CAD build for the part. Positions are in the model's coordinates, mm. Face numbers are marked on the shaded views. A direction names the side the tool comes from. Coordinates: 2 decimals unless noted, no trailing zeros. Loops run counter-clockwise (first coordinate to the right, second up) from the corner with the lowest first, then second, coordinate; pieces in that order, holes last. Notation, with made-up numbers: M 29.25,-15.75 L 37.25,-15.75 A28 cw 37.25,11.25 Z; hole C 65.5,66.25 d4. An arc over 180 degrees is marked long. Answer as a JSON object with one key per item and string values. Group by question number.
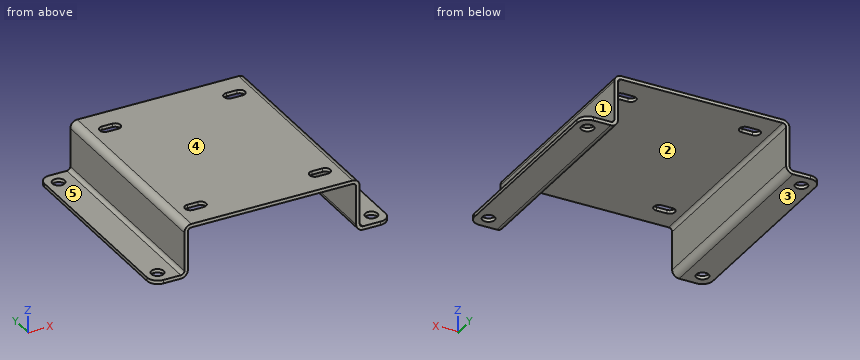
Autodesk Inventor part; units mm, degrees
ref_plane "YZ Plane" through (0, 0, 0) normal (1, 0, 0) x (0, 1, 0)
ref_plane "XZ Plane" through (0, 0, 0) normal (0, 1, 0) x (-1, 0, 0)
ref_plane "XY Plane" through (0, 0, 0) normal (0, 0, 1) x (1, 0, 0)
sketch "Sketch1" plane through (0, 0, 0) normal (0, 0, 1) x (1, 0, 0)
  line L0 (-50, -60) -> (50, -60)
  line L1 (50, -60) -> (50, 60)
  line L2 (50, 60) -> (-50, 60)
  line L3 (-50, 60) -> (-50, -60)
  line L4 (-50, -60) -> (50, 60) construction
  line L5 (50, -60) -> (-50, 60) construction
  point P0 (0, 0)
  dimension "d0" = 100
  dimension "d1" = 120
extrude "Plate1" add sketch "Sketch1" along normal blind 2
sketch "Sketch5" plane through (48, -60, 2) normal (1, 0, 0) x (0, 1, 0)
  line L0 (120, 0) -> (0, 0)
  line L1 (0, 0) -> (0, -30)
  line L2 (0, -30) -> (120, -30)
  line L3 (120, -30) -> (120, 0)
edge flange "Flange2" height 30 angle 90 thickness 2 bend radius 2 thickness toward (1, 0, 0) relief tear relief width 2 relief depth 1 corner gap 2 corner form 0 edges at (50, 0, 0) (-50, 0, 0) wall of the first edge with corners at (48, 60, 2) (48, -60, 2) (48, -60, -28) (48, 60, -28)
bend "Bend2"
corner "Corner2"
sketch "Sketch6" plane through (-48, -60, -26) normal (0, 0, -1) x (-1, 0, 0)
  line L0 (0, 120) -> (0, 0)
  line L1 (0, 0) -> (20, 0)
  line L2 (20, 0) -> (20, 120)
  line L3 (20, 120) -> (0, 120)
edge flange "Flange3" height 20 angle 90 thickness 2 bend radius 2 thickness toward (0, 0, -1) relief tear relief width 2 relief depth 1 corner gap 2 corner form 0 edges at (-50, 0, -28) (50, 0, -28) wall of the first edge with corners at (-48, 60, -26) (-48, -60, -26) (-68, -60, -26) (-68, 60, -26)
bend "Bend3"
corner "Corner3"
sketch "Sketch7" plane through (0, 0, 2) normal (0, 0, 1) x (1, 0, 0)
  line L0 (-38.5, 45) -> (-32.5, 45) construction
  line L1 (-38.5, 48) -> (-32.5, 48)
  line L2 (-32.5, 42) -> (-38.5, 42)
  arc A0 (-38.5, 48) -> (-38.5, 42) centre (-38.5, 45) ccw
  arc A1 (-32.5, 42) -> (-32.5, 48) centre (-32.5, 45) ccw
  line L3 (0, 0) -> (0, 36.7508)
  line L4 (0, 0) -> (-25.7119, 0)
  line L5 (32.5, 45) -> (38.5, 45) construction
  line L6 (32.5, 48) -> (38.5, 48)
  line L7 (38.5, 42) -> (32.5, 42)
  arc A2 (32.5, 48) -> (32.5, 42) centre (32.5, 45) ccw
  arc A3 (38.5, 42) -> (38.5, 48) centre (38.5, 45) ccw
  line L8 (-38.5, -45) -> (-32.5, -45) construction
  line L9 (-38.5, -42) -> (-32.5, -42)
  line L10 (-32.5, -48) -> (-38.5, -48)
  arc A4 (-38.5, -42) -> (-38.5, -48) centre (-38.5, -45) ccw
  arc A5 (-32.5, -48) -> (-32.5, -42) centre (-32.5, -45) ccw
  line L11 (32.5, -45) -> (38.5, -45) construction
  line L12 (32.5, -42) -> (38.5, -42)
  line L13 (38.5, -48) -> (32.5, -48)
  arc A6 (32.5, -42) -> (32.5, -48) centre (32.5, -45) ccw
  arc A7 (38.5, -48) -> (38.5, -42) centre (38.5, -45) ccw
  point P0 (-35.5, 45)
  point P1 (35.5, 45)
  point P2 (-35.5, -45)
  point P3 (35.5, -45)
  dimension "d42" = 6
  dimension "d43" = 6
  dimension "d50" = 71
  dimension "d51" = 90
extrude "Cut1" cut sketch "Sketch7" against normal blind 2
sketch "Sketch8" plane through (-68, -60, -26) normal (0, 0, 1) x (1, 0, 0)
  circle A0 centre (7, 112) radius 3.5
  circle A1 centre (7, 8) radius 3.5
  line L0 (16, 120) -> (0, 120)
  line L1 (0, 120) -> (0, 0)
  line L2 (0, 60) -> (53.6667, 60)
  point P0 (68, 60)
  dimension "d54" = 7
  dimension "d55" = 8
  dimension "d56" = 7
extrude "Cut2" cut sketch "Sketch8" against normal blind 2
mirror "Mirror1" about plane through (0, 0, 0) normal (1, 0, 0) of "Cut2"
fillet "Corner Round1" radius 6 4 edges at (-68, -60, -27) (-68, 60, -27) (68, 60, -27) (68, -60, -27)
equation "\"d52\" = Thickness"
equation "\"d57\" = Thickness"
equation "\"d2\" = Thickness"
equation "\"d22\" = BendReliefWidth"
equation "\"d23\" = BendReliefDepth"
equation "\"d24\" = MinimumRemnant"
equation "\"d25\" = TransitionRadius"
equation "\"d28\" = BendRadius"
equation "\"d29\" = CornerReliefSize"
equation "\"d30\" = GapSize"
equation "\"d31\" = JacobiRadiusSize"
equation "\"d32\" = BendReliefWidth"
equation "\"d33\" = BendReliefDepth"
equation "\"d34\" = MinimumRemnant"
equation "\"d35\" = TransitionRadius"
equation "\"d38\" = BendRadius"
equation "\"d39\" = CornerReliefSize"
equation "\"d40\" = GapSize"
equation "\"d41\" = JacobiRadiusSize"
equation "\"BendRadius\" = Thickness"
equation "\"BendReliefWidth\" = Thickness"
equation "\"BendReliefDepth\" = 0.5 * Thickness"
equation "\"CornerReliefSize\" = 4 * Thickness"
equation "\"MinimumRemnant\" = 2 * Thickness"
equation "\"TransitionRadius\" = BendRadius"
equation "\"JacobiRadiusSize\" = BendRadius"
equation "\"GapSize\" = Thickness"
properties part number "PNS- motor 030 reductor pillar"
Item 1: Pin check, flat tips, straight feed: pin 1 (8 mm diameter, centred on y = -2, z = -12.5, fed in from +X); pin 2 (4 mm diameter, centred on x = 34.5, z = -2.5, fed in from +Y); pin 3 (5 mm diameter, centred on x = 63, y = 28.5, fed in from +Z); pin 4 (11 mm diameter, centred on y = -5, z = -16.5, fed in from -X). Stop position of each tip, or through.
Item 2: Tool access for the marked faces 1, 2, 3, 4 and 5: list every direction of +Z, -Z, +X, -X, +Y, -Y with a clear straight run to the whole face (end or side of a thin tool).
Item 3: Slice it at A-A, the plane x = 35. Write the cut outline in (y, z), then the cut area to 3 significant figures.
Item 4: Slice it at B-B, the plane y = -52. Write the cut outline in (x, z).
Item 5: Drill centre lines: L1, parallel to Y at x = -61, z = -26.35; L2, parallel to X at y = 45, z = -16.5; L3, parallel to Z at x = 7.5, y = -23. Where is each one in solid material? Low to high. Write a range as from..to.
Item 6: Slice it at C-C, the plane z = -16. Write the cut outline in (x, y).
Item 7: Slice it at D-D, the plane y = 13. Write the cut outline in (x, z).
Computed:
{
 "1": {"pin 1": "x = 50", "pin 2": "through", "pin 3": "z = -26", "pin 4": "x = -50"},
 "2": {"face 1": "+Z, +X, +Y, -Y", "face 2": "-Z, +Y, -Y", "face 3": "-Z, +X, -X, +Y, -Y", "face 4": "+Z, +X, -X, +Y, -Y", "face 5": "+Z, -X, +Y, -Y"},
 "3": {"outline": "M -60,0 L -48,0 L -48,2 L -60,2 Z; M -42,0 L 42,0 L 42,2 L -42,2 Z; M 48,0 L 60,0 L 60,2 L 48,2 Z", "area": "216 mm2"},
 "4": {"outline": "M -68,-28 L -64.5,-28 L -64.5,-26 L -68,-26 Z; M -57.5,-28 L -52,-28 A4 ccw -48,-24 L -48,-2 A2 cw -46,0 L 46,0 A2 cw 48,-2 L 48,-24 A4 ccw 52,-28 L 57.5,-28 L 57.5,-26 L 52,-26 A2 cw 50,-24 L 50,-2 A4 ccw 46,2 L -46,2 A4 ccw -50,-2 L -50,-24 A2 cw -52,-26 L -57.5,-26 Z; M 64.5,-28 L 68,-28 L 68,-26 L 64.5,-26 Z"},
 "5": {"L1": "-60..-55.5, -48.5..48.5, 55.5..60", "L2": "-50..-48, 48..50", "L3": "0..2"},
 "6": {"outline": "M -50,-60 L -48,-60 L -48,60 L -50,60 Z; M 48,-60 L 50,-60 L 50,60 L 48,60 Z"},
 "7": {"outline": "M -68,-28 L -52,-28 A4 ccw -48,-24 L -48,-2 A2 cw -46,0 L 46,0 A2 cw 48,-2 L 48,-24 A4 ccw 52,-28 L 68,-28 L 68,-26 L 52,-26 A2 cw 50,-24 L 50,-2 A4 ccw 46,2 L -46,2 A4 ccw -50,-2 L -50,-24 A2 cw -52,-26 L -68,-26 Z"}
}
